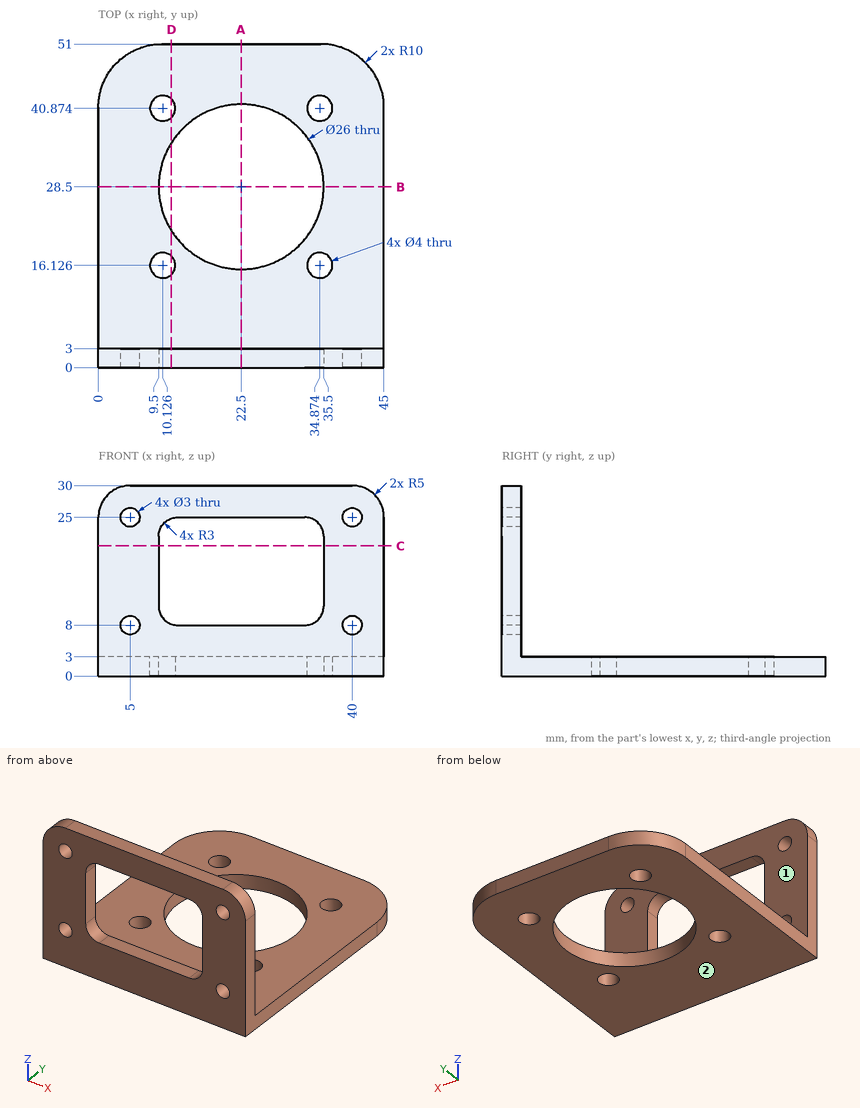
Part print with two shaded views. Sizes in mm from the minimum x, y, z corner. A direction names the side the tool comes from. Round coordinates to 2 decimals unless told otherwise and drop trailing zeros. Order: outer loops, then holes, each group sorted by start corner. A loop starts at its lowest first (then second) coordinate and runs counter-clockwise, first axis right, second up. Notation, with made-up numbers: (69.25, 36.25) - (82.25, 36.25) arc R17 cw to (82.25, 62.25) - close; hole circle Ø3 at (52.25, -5.75). An arc over 180 degrees is marked (long way). Answer in a Markdown table with one row per item. Add a question column.
(1) Probe L1, parallel to Z at x = 40, y = 0.7; L2, parallel to Z at x = 5, y = 22. List the from-to ranges inside material, lowest first. Write a range as [from, to].
(2) Band-saw the part on A-A on x = 22.5. List the corners of the cut face in (y, z).
(3) Drop flat-ended pins along their axis: pin 1 Ø3.5 at (x, z) = (40, 8) entering from +Y; pin 2 Ø4.5 at (x, y) = (34.87, 16.13) entering from +Z. Give the stop position or say it passes through.
(4) Band-saw the part on B-B on y = 28.5. List the corners of the cut face in (x, z), and give its area (3 significant figures).
(5) Band-saw the part on D-D on x = 11.5. List the corners of the cut face in (y, z), and give its area (3 significant figures).
(6) 3-axis set-ups, long thin cutter, end or side, ignore diameter. For the marked faces 1 and 2: which of +Z, -Z, +X, -X, +Y, -Y reach the whole face in a straight line?
Data:
| question | item | result |
|---|---|---|
| 1 | L1 | z = [0, 6.5], [9.5, 23.5], [26.5, 30] |
| 1 | L2 | z = [0, 3] |
| 2 | outline | (0, 0) - (15.5, 0) - (15.5, 3) - (3, 3) - (3, 8) - (0, 8) - close; (0, 25) - (3, 25) - (3, 30) - (0, 30) - close; (41.5, 0) - (51, 0) - (51, 3) - (41.5, 3) - close |
| 3 | pin 1 | stops at y = 3 |
| 3 | pin 2 | stops at z = 3 |
| 4 | outline | (0, 0) - (9.5, 0) - (9.5, 3) - (0, 3) - close; (35.5, 0) - (45, 0) - (45, 3) - (35.5, 3) - close |
| 4 | area | 57.0 mm^2 |
| 5 | outline | (0, 0) - (14.67, 0) - (14.67, 3) - (3, 3) - (3, 8.17) - (0, 8.17) - close; (0, 24.83) - (3, 24.83) - (3, 30) - (0, 30) - close; (17.58, 0) - (21.57, 0) - (21.57, 3) - (17.58, 3) - close; (35.43, 0) - (39.42, 0) - (39.42, 3) - (35.43, 3) - close; (42.33, 0) - (51, 0) - (51, 3) - (42.33, 3) - close |
| 5 | area | 125 mm^2 |
| 6 | face 1 | +Z, +X, -X, +Y |
| 6 | face 2 | -Z, +X, -X, +Y, -Y |
